from build123d import *

# Parameters (mm, degrees)
F1_DEPTH = 304.8


with BuildPart() as f1:
    # F0 (on Right) → F1 (new body)
    with BuildSketch(Plane.YZ):
        with BuildLine():
            Line((0, 0), (0, 50.8))
            Line((0, 50.8), (-47.36958, 50.8))
            Line((-47.36958, 50.8), (-47.36958, 47.071686))
            ThreePointArc((-47.36958, 47.071686), (-46.642815, 45.05011), (-44.795237, 43.954021))
            Line((-44.795237, 43.954021), (-14.673686, 38.150726))
            ThreePointArc((-14.673686, 38.150726), (-10.978529, 35.958548), (-9.525, 31.915396))
            Line((-9.525, 31.915396), (-9.525, 0))
            Line((-9.525, 0), (-9.525, -31.915396))
            ThreePointArc((-9.525, -31.915396), (-10.978529, -35.958548), (-14.673686, -38.150726))
            Line((-14.673686, -38.150726), (-44.795237, -43.954021))
            ThreePointArc((-44.795237, -43.954021), (-46.642815, -45.05011), (-47.36958, -47.071686))
            Line((-47.36958, -47.071686), (-47.36958, -50.8))
            Line((-47.36958, -50.8), (0, -50.8))
            Line((0, -50.8), (0, 0))
        make_face()
    extrude(amount=F1_DEPTH)


solid = f1.part
Build history of the part. All positions in model axes, mm. A direction names the side the tool comes from. Round coordinates to 2 decimals unless told otherwise and drop trailing zeros. Write each loop counter-clockwise with the first axis right and the second up, starting at its lowest first coordinate (ties: lowest second). Pieces come first, ordered by that corner, then holes. Notation, with made-up numbers: M 4.5,-39.75 L 41.5,-39.75 A20 ccw 41.5,-0.75 Z; hole C 72,-32.5 d6. An arc over 180 degrees is marked long. Use CSV: the item, a comma, the result in double quotes.
1. Wall check: probe 1 along Y at (x, z) = (265.5, -32.5); probe 2 along Z at (x, y) = (124.5, -14.5); probe 3 along Z at (x, y) = (281.5, -44.5). Give the ranges that are in metal, low to high. Write a range as from..to.
Reply:
probe 1,"y = -9.55..0"
probe 2,"z = -50.8..-38.11, 38.11..50.8"
probe 3,"z = -50.8..-43.9, 43.9..50.8"
2. Saw through at D-D (y = -22). Give the cut face in (x, z), plus the area to 3 significant figures.
Reply:
outline,"M 0,-50.8 L 304.8,-50.8 L 304.8,-39.56 L 0,-39.56 Z; M 0,39.56 L 304.8,39.56 L 304.8,50.8 L 0,50.8 Z"
area,"6,850 mm²"
3. Two-plate mould, pull along Z, no slides. Class faces 3 (the face through (150, -24, -50.8)), 4 (the face through (150, 0, -1)), 5 (the face through (150.27, -11.02, 36.01)), 6 (the face through (150.266, -29.945, 41.093)): +Z half, -Z half, draft (parallel to the pull), parting line (faces both ways), or undercut.
Reply:
face 3,"-Z half"
face 4,"draft"
face 5,"undercut"
face 6,"undercut"
4. Tool access for faces 1 (the face through (150.27, -29.52, -41.01)), 2 (the face through (150, -23, 50.8)): list every direction of +Z, -Z, +X, -X, +Y, -Y with a clear straight run to the whole face (end or side of a thin tool).
Reply:
face 1,"+X, -X, -Y"
face 2,"+Z, +X, -X, +Y, -Y"
5. Flat gauge pins, fed straight in: pin 1 (5 mm diameter, centred on x = 39, z = 9, fed in from -Y) (3 decimals); pin 2 (2 mm diameter, centred on y = -11.5, z = -29.5, fed in from +X). Where does each tip first touch, or does it go through?
Reply:
pin 1,"stops at y = -9.525"
pin 2,"passes through"
6. Saw through at C-C (z = -24.5). Give the cut face in (x, y) (3 decimals), plus the area to 3 significant figures.
Reply:
outline,"M 0,-9.525 L 304.8,-9.525 L 304.8,0 L 0,0 Z"
area,"2,900 mm²"
7. Saw through at A-A (y = -38). Give the cut face in (x, z).
Reply:
outline,"M 0,-50.8 L 304.8,-50.8 L 304.8,-42.64 L 0,-42.64 Z; M 0,42.64 L 304.8,42.64 L 304.8,50.8 L 0,50.8 Z"
8. Saw through at B-B (x = 97). Give the cut face in (y, z) (3 decimals).
Reply:
outline,"M -47.37,-50.8 L 0,-50.8 L 0,50.8 L -47.37,50.8 L -47.37,47.072 A3.175 ccw -44.795,43.954 L -14.674,38.151 A6.35 cw -9.525,31.915 L -9.525,-31.915 A6.35 cw -14.674,-38.151 L -44.795,-43.954 A3.175 ccw -47.37,-47.072 Z"
